Build history of the part. All positions in model axes, mm. Face numbers are marked on the shaded views. Round coordinates to 2 decimals unless told otherwise and drop trailing zeros. Write each loop counter-clockwise with the first axis right and the second up, starting at its lowest first coordinate (ties: lowest second). Pieces come first, ordered by that corner, then holes. Notation, with made-up numbers: (-8, -1.5) -> (25, -1.5) arc R16 cw to (25, 12.5) -> close; hole circle Ø11 at (-19.75, 0.5). An arc over 180 degrees is marked (long way). Return JSON: item names as keys, results as strings.
from build123d import *

# Parameters (mm, degrees)
BOSS_EXTRUDE1_DEPTH     = 18
CUT_EXTRUDE2_DEPTH      = 9
CUT_EXTRUDE3_DEPTH      = 30.344292319
CUT_EXTRUDE3_DEPTH_BACK = 12.5
SKETCH6_6_W             = 12.6
SKETCH6_6_H             = 5.1
CUT_EXTRUDE4_DEPTH      = 2.5
CHAMFER1_SIZE           = 10
CHAMFER1_SIZE2          = 5.773502692
CHAMFER2_SIZE           = 1
CUT_EXTRUDE5_START      = -12.5
CUT_EXTRUDE5_DEPTH      = 17.844292319


with BuildPart() as part:
    # Sketch1 → Boss-Extrude1 (new body)
    with BuildSketch(Plane(origin=(0, 0, 0), x_dir=(1, 0, 0), z_dir=(0, 1, 0))):
        Polygon((0, 0), (0, -34), (34, 0), align=None)
    extrude(amount=BOSS_EXTRUDE1_DEPTH)

    # Sketch6 → Cut-Extrude2 (cut)
    # profile 1 of 8: a face of its own
    with BuildSketch(Plane(origin=(15.196708808, 12.408060783, 15.196708808), x_dir=(0.7071067811865475, 0, -0.7071067811865476), z_dir=(0.6123724356957942, 0.5000000000000011, 0.6123724356957941))):
        Polygon((-24.04163056, 7.366311807), (-24.04163056, -5.100477721), (24.04163056, -5.100477721), (24.04163056, 7.366311807), (-8.989412587, 7.366311807), (-14.222807352, -3.100477721), (0, -3.100477721), (0, -4.100477721), (-20.312977295, -4.100477721), (-14.579582531, 7.366311807), align=None)
        with BuildLine():
            ThreePointArc((2.248888614, -1.100477721), (0, -1.950477721), (-2.248888614, -1.100477721))
            Line((-2.248888614, -1.100477721), (-6.3, -1.100477721))
            Line((-6.3, -1.100477721), (-6.3, 3.999522279))
            Line((-6.3, 3.999522279), (-2.248888614, 3.999522279))
            ThreePointArc((-2.248888614, 3.999522279), (0, 4.849522279), (2.248888614, 3.999522279))
            Line((2.248888614, 3.999522279), (6.3, 3.999522279))
            Line((6.3, 3.999522279), (6.3, -1.100477721))
            Line((6.3, -1.100477721), (2.248888614, -1.100477721))
        make_face(mode=Mode.SUBTRACT)
    # profile 2 of 8: a face of its own
    with BuildSketch(Plane(origin=(15.196708808, 12.408060783, 15.196708808), x_dir=(0.7071067811865475, 0, -0.7071067811865476), z_dir=(0.6123724356957942, 0.5000000000000011, 0.6123724356957941))):
        with BuildLine():
            ThreePointArc((3.4, 1.449522279), (3.098888614, 0.050633664), (2.248888614, -1.100477721))
            Line((2.248888614, -1.100477721), (6.3, -1.100477721))
            Line((6.3, -1.100477721), (6.3, 3.999522279))
            Line((6.3, 3.999522279), (2.248888614, 3.999522279))
            ThreePointArc((2.248888614, 3.999522279), (3.098888614, 2.848410893), (3.4, 1.449522279))
        make_face()
    # profile 3 of 8: a face of its own
    with BuildSketch(Plane(origin=(15.196708808, 12.408060783, 15.196708808), x_dir=(0.7071067811865475, 0, -0.7071067811865476), z_dir=(0.6123724356957942, 0.5000000000000011, 0.6123724356957941))):
        with BuildLine():
            Line((-6.3, -1.100477721), (-2.248888614, -1.100477721))
            ThreePointArc((-2.248888614, -1.100477721), (-3.4, 1.449522279), (-2.248888614, 3.999522279))
            Line((-2.248888614, 3.999522279), (-6.3, 3.999522279))
            Line((-6.3, 3.999522279), (-6.3, -1.100477721))
        make_face()
    # profile 4 of 8: a face of its own
    with BuildSketch(Plane(origin=(15.196708808, 12.408060783, 15.196708808), x_dir=(0.7071067811865475, 0, -0.7071067811865476), z_dir=(0.6123724356957942, 0.5000000000000011, 0.6123724356957941))):
        with BuildLine():
            Line((0, -1.100477721), (-2.248888614, -1.100477721))
            ThreePointArc((-2.248888614, -1.100477721), (0, -1.950477721), (2.248888614, -1.100477721))
            Line((2.248888614, -1.100477721), (0, -1.100477721))
        make_face()
    # profile 5 of 8: a face of its own
    with BuildSketch(Plane(origin=(15.196708808, 12.408060783, 15.196708808), x_dir=(0.7071067811865475, 0, -0.7071067811865476), z_dir=(0.6123724356957942, 0.5000000000000011, 0.6123724356957941))):
        with BuildLine():
            ThreePointArc((2.248888614, 3.999522279), (0, 4.849522279), (-2.248888614, 3.999522279))
            Line((-2.248888614, 3.999522279), (0, 3.999522279))
            Line((0, 3.999522279), (2.248888614, 3.999522279))
        make_face()
    # profile 6 of 8: a face of its own
    with BuildSketch(Plane(origin=(15.196708808, 12.408060783, 15.196708808), x_dir=(0.7071067811865475, 0, -0.7071067811865476), z_dir=(0.6123724356957942, 0.5000000000000011, 0.6123724356957941))):
        with BuildLine():
            ThreePointArc((-2.248888614, 3.999522279), (-3.4, 1.449522279), (-2.248888614, -1.100477721))
            Line((-2.248888614, -1.100477721), (0, -1.100477721))
            Line((0, -1.100477721), (2.248888614, -1.100477721))
            ThreePointArc((2.248888614, -1.100477721), (3.098888614, 0.050633664), (3.4, 1.449522279))
            ThreePointArc((3.4, 1.449522279), (3.098888614, 2.848410893), (2.248888614, 3.999522279))
            Line((2.248888614, 3.999522279), (0, 3.999522279))
            Line((0, 3.999522279), (-2.248888614, 3.999522279))
        make_face()
    # profile 7 of 8: a face of its own
    with BuildSketch(Plane(origin=(15.196708808, 12.408060783, 15.196708808), x_dir=(0.7071067811865475, 0, -0.7071067811865476), z_dir=(0.6123724356957942, 0.5000000000000011, 0.6123724356957941))):
        Polygon((-12.902531548, 7.366311807), (-14.579582531, 7.366311807), (-20.312977295, -4.100477721), (0, -4.100477721), (0, -3.100477721), (-14.222807352, -3.100477721), (-8.989412587, 7.366311807), (-10.666463571, 7.366311807), (-15.899858335, -3.100477721), (-18.135926312, -3.100477721), align=None)
    # profile 8 of 8: a face of its own
    with BuildSketch(Plane(origin=(15.196708808, 12.408060783, 15.196708808), x_dir=(0.7071067811865475, 0, -0.7071067811865476), z_dir=(0.6123724356957942, 0.5000000000000011, 0.6123724356957941))):
        Polygon((-10.666463571, 7.366311807), (-12.902531548, 7.366311807), (-18.135926312, -3.100477721), (-15.899858335, -3.100477721), align=None)
    extrude(amount=CUT_EXTRUDE2_DEPTH, mode=Mode.SUBTRACT)

    # Sketch6<6> → Cut-Extrude3 (cut, two sides: drawn at the far end of the back side and taken through both)
    with BuildSketch(Plane(origin=(15.196708808, 12.408060783, 15.196708808), x_dir=(0.7071067811865475, 0, -0.7071067811865476), z_dir=(0.6123724356957942, 0.5000000000000011, 0.6123724356957941)).offset(-CUT_EXTRUDE3_DEPTH_BACK)):
        with Locations((0, 1.449522279)):
            Rectangle(SKETCH6_6_W, SKETCH6_6_H)
    extrude(amount=CUT_EXTRUDE3_DEPTH + CUT_EXTRUDE3_DEPTH_BACK, mode=Mode.SUBTRACT)

    # Sketch6<8> → Cut-Extrude4 (cut)
    with BuildSketch(Plane(origin=(15.196708808, 12.408060783, 15.196708808), x_dir=(0.7071067811865475, 0, -0.7071067811865476), z_dir=(0.6123724356957942, 0.5000000000000011, 0.6123724356957941))):
        Polygon((-12.902531548, 7.366311807), (-14.579582531, 7.366311807), (-20.312977295, -4.100477721), (0, -4.100477721), (0, -3.100477721), (-14.222807352, -3.100477721), (-8.989412587, 7.366311807), (-10.666463571, 7.366311807), (-15.899858335, -3.100477721), (-18.135926312, -3.100477721), align=None)
    cut_extrude4 = extrude(amount=-CUT_EXTRUDE4_DEPTH, mode=Mode.SUBTRACT)

    # Mirror1: Cut-Extrude4 across plane
    add(cut_extrude4.mirror(Plane(origin=(0, 0, 0), x_dir=(0.7071067811865476, 0, 0.7071067811865476), z_dir=(-0.7071067811865477, 0, 0.7071067811865475))), mode=Mode.SUBTRACT)

    # Chamfer1
    chamfer1_edges = [part.edges().sort_by_distance(p)[0] for p in [
        (17, 0, 17),
    ]]
    chamfer1_side = [part.faces().sort_by_distance(p)[0] for p in [
        (11.333333333, 0, 11.333333333),
    ]]
    chamfer(chamfer1_edges, length=CHAMFER1_SIZE, length2=CHAMFER1_SIZE2, reference=chamfer1_side[0])

    # Chamfer2
    chamfer2_edges = [part.edges().sort_by_distance(p)[0] for p in [
        (19.138998013, 13.6633839, 10.22945257),
        (15.585786438, 11.45501912, 15.585786438),
        (10.22945257, 13.6633839, 19.138998013),
        (13.782664146, 15.871748679, 13.782664146),
    ]]
    chamfer(chamfer2_edges, length=CHAMFER2_SIZE)

    # Sketch6<9> → Cut-Extrude5 (cut, through all)
    with BuildSketch(Plane(origin=(15.196708808, 12.408060783, 15.196708808), x_dir=(0.7071067811865475, 0, -0.7071067811865476), z_dir=(0.6123724356957942, 0.5000000000000011, 0.6123724356957941)).offset(CUT_EXTRUDE5_START)):
        with BuildLine():
            ThreePointArc((2.248888614, 3.999522279), (0, 4.849522279), (-2.248888614, 3.999522279))
            Line((-2.248888614, 3.999522279), (0, 3.999522279))
            Line((0, 3.999522279), (2.248888614, 3.999522279))
        make_face()
        with BuildLine():
            ThreePointArc((-2.248888614, 3.999522279), (-3.4, 1.449522279), (-2.248888614, -1.100477721))
            Line((-2.248888614, -1.100477721), (0, -1.100477721))
            Line((0, -1.100477721), (2.248888614, -1.100477721))
            ThreePointArc((2.248888614, -1.100477721), (3.098888614, 0.050633664), (3.4, 1.449522279))
            ThreePointArc((3.4, 1.449522279), (3.098888614, 2.848410893), (2.248888614, 3.999522279))
            Line((2.248888614, 3.999522279), (0, 3.999522279))
            Line((0, 3.999522279), (-2.248888614, 3.999522279))
        make_face()
        with BuildLine():
            Line((0, -1.100477721), (-2.248888614, -1.100477721))
            ThreePointArc((-2.248888614, -1.100477721), (0, -1.950477721), (2.248888614, -1.100477721))
            Line((2.248888614, -1.100477721), (0, -1.100477721))
        make_face()
    extrude(amount=-CUT_EXTRUDE5_DEPTH, mode=Mode.SUBTRACT)


solid = part.part
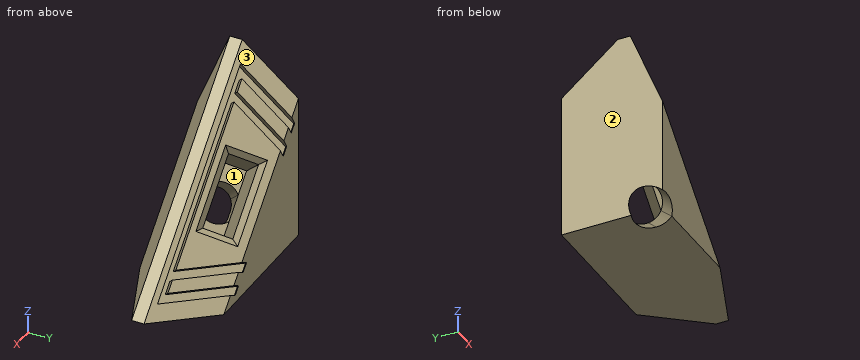
Q1. Two-plate mould, pull along Z, no slides. Class the marked faces 1, 2 and 3: +Z half, -Z half, draft (parallel to the pull), parting line (faces both ways), or undercut.
Verdict:
{"face 1": "undercut", "face 2": "draft", "face 3": "+Z half"}
Q2. Saw through at C-C on z = 24. List the corners of the cut face in (x, y).
Verdict:
{"outline": "(0, 1.69) -> (10, 5.77) -> (10, 7.99) -> (9.29, 8.86) -> (6.23, 7.61) -> (5.52, 8.47) -> (8.59, 9.72) -> (6.24, 12.6) -> (4.7, 9.48) -> (3.52, 10.93) -> (5.05, 14.05) -> (3.47, 15.99) -> (1.94, 12.86) -> (0.75, 14.32) -> (2.28, 17.44) -> (1.83, 18) -> (0, 18) -> close"}
Q3. Saw through at D-D on x = 11.5. List the corners of the cut face in (y, z).
Verdict:
{"outline": "(0, 0) -> (18, 0) -> (18, 14.33) -> (16.74, 15.36) -> (15.37, 14.84) -> (10.37, 2.59) -> (7.38, 2.59) -> (5.21, 4.36) -> (10.96, 18.45) -> (10.59, 20.38) -> (9.72, 21.09) -> (8.47, 18.02) -> (7.61, 18.73) -> (8.86, 21.79) -> (7.99, 22.5) -> (5.77, 22.5) -> (0, 8.36) -> close"}
Q4. Pin check, flat tips, straight feed: pin 1 Ø4 at (x, z) = (15, 12.5) entering from -Y; pin 2 Ø6 at (x, z) = (11.5, 26.5) entering from +Y. Stop position of each tip, or through.
Verdict:
{"pin 1": "stops at y = 1.97", "pin 2": "stops at y = 8.29"}
Q5. Saw through at A-A on x = 28.5. List the corners of the cut face in (y, z).
Verdict:
{"outline": "(3.53, 0) -> (14.73, 0) -> (11.93, 2.28) -> (8.81, 0.75) -> (7.61, 1.73) -> (8.86, 4.79) -> (7.99, 5.5) -> (5.77, 5.5) -> close; (9.22, 2.85) -> (10.48, 3.47) -> (9.72, 4.09) -> close"}
Q6. Wall check: L1, parallel to Z at x = 15.5, y = 4.5; L2, parallel to Y at x = 4.5, z = 8.5; L3, parallel to Y at x = 12, z = 6.5. Give the ranges that are in metal, low to high.
Verdict:
{"L1": "z = 0 to 15.38", "L2": "y = 0 to 4.8, 9.93 to 18", "L3": "y = 0 to 6.28, 12.17 to 18"}
Q7. Saw through at B-B on y = 12.5. List the corners of the cut face in (x, z), then the cut area to 3 significant figures.
Verdict:
{"outline": "(0, 0) -> (30.32, 0) -> (28.04, 2.28) -> (25.48, 0.75) -> (24.3, 1.94) -> (26.85, 3.47) -> (25.27, 5.05) -> (22.72, 3.52) -> (21.53, 4.7) -> (24.08, 6.24) -> (20.32, 10) -> (18.8, 9.89) -> (14.11, 5.2) -> (5.2, 14.11) -> (9.89, 18.8) -> (10, 20.32) -> (6.24, 24.08) -> (4.7, 21.53) -> (3.52, 22.72) -> (5.05, 25.27) -> (3.47, 26.85) -> (1.94, 24.3) -> (0.75, 25.48) -> (2.28, 28.04) -> (0, 30.32) -> close", "area": "341 mm²"}
